Build history of the part. All positions in model axes, mm. Face numbers are marked on the shaded views. A direction names the side the tool comes from. Coordinates: 2 decimals unless noted, no trailing zeros. Order: outer loops, then holes, each group sorted by start corner. A loop starts at its lowest first (then second) coordinate and runs counter-clockwise, first axis right, second up. Notation, with made-up numbers: (76.5, 38) - (135.5, 38) arc R30 ccw to (135.5, 62) - close; hole circle Ø5 at (18, -12.75). An arc over 180 degrees is marked (long way). Write each question's results on one line, items separated by ' | '.
from build123d import *

# Parameters (mm, degrees)
SKETCH1_R               = 70
BOSS_EXTRUDE1_DEPTH     = 35
SKETCH2_R               = 62.5
BOSS_EXTRUDE2_DEPTH     = 150
FILLET1_R               = 20
SKETCH3_R               = 57.5
BOSS_EXTRUDE3_DEPTH     = 325
CUT_EXTRUDE1_DEPTH      = 15
CUT_EXTRUDE1_DEPTH_BACK = 15
FILLET2_R               = 10


with BuildPart() as part:
    # Sketch1 → Boss-Extrude1 (new body)
    with BuildSketch(Plane.XY):
        Circle(SKETCH1_R)
    extrude(amount=BOSS_EXTRUDE1_DEPTH)

    # Sketch2 → Boss-Extrude2 (add)
    with BuildSketch(Plane.XY):
        Circle(SKETCH2_R)
    extrude(amount=-BOSS_EXTRUDE2_DEPTH)

    # Fillet1
    # the kernel refuses this fillet: 20 mm, written as the material it adds along each edge
    with BuildSketch(Plane(origin=(0, 0, 0), x_dir=(1, 0, 0), z_dir=(0, -1, 0))) as fillet1_piece_1:
        with BuildLine():
            CenterArc((82.5, -15.612494996), FILLET1_R, 128.682187453, 51.317812547)
            Line((62.5, -15.612494996), (62.1, -15.612494996))
            Line((62.1, -15.612494996), (62.1, 0))
            Line((62.1, 0), (62.5, 0.4))
            ThreePointArc((62.5, 0.4), (66.25, 0.4), (69.75, 0.3122499))
            Line((69.75, 0.3122499), (70, 0))
        make_face()
    revolve(axis=Axis((0, 0, 0), (0, 0, 1)))

    # Sketch3 → Boss-Extrude3 (add)
    with BuildSketch(Plane.XY):
        Circle(SKETCH3_R)
    extrude(amount=BOSS_EXTRUDE3_DEPTH)

    # Sketch4 → Cut-Extrude1 (cut, two sides: drawn at the far end of the back side and taken through both)
    with BuildSketch(Plane(origin=(0, 0, 0), x_dir=(0, 0, -1), z_dir=(1, 0, 0)).offset(-CUT_EXTRUDE1_DEPTH_BACK)):
        Polygon((-240, 0), (-251.375, 273), (-60, 273), (-60, 0), (-60, -273), (-228.625, -273), align=None)
    extrude(amount=CUT_EXTRUDE1_DEPTH + CUT_EXTRUDE1_DEPTH_BACK, mode=Mode.SUBTRACT)

    # Fillet2
    fillet2_edges = [part.edges().sort_by_distance(p)[0] for p in [
        (-62.5, 0, -150),
    ]]
    fillet(fillet2_edges, radius=FILLET2_R)


solid = part.part
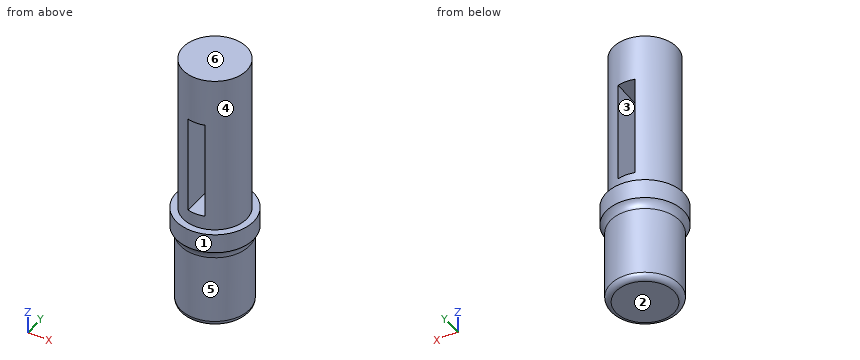
1. Band-saw the part on A-A on y = 0. Give the cut face in (x, z), then the cut area to 3 significant figures.
Solved:
outline: (-70, 0) arc R20 cw to (-62.5, -15.61) - (-62.5, -140) arc R10 ccw to (-52.5, -150) - (52.5, -150) arc R10 ccw to (62.5, -140) - (62.5, -15.61) arc R20 cw to (70, 0) - (70, 35) - (57.5, 35) - (57.5, 325) - (-57.5, 325) - (-57.5, 35) - (-70, 35) - close; hole (-15, 60) - (15, 60) - (15, 240) - (-15, 240) - close | area: 51,600 mm2
2. Band-saw the part on C-C on z = 206. Give the cut face in (x, y).
Solved:
outline: (-15, -55.51) - (-15, 55.51) arc R57.5 ccw to start; (15, -55.51) arc R57.5 ccw to (15, 55.51) - close
3. Two-plate mould, pull along X, no slides. Class the marked faces 1, 2 and 3: +X half, -X half, draft (parallel to the pull), parting line (faces both ways), or undercut.
Solved:
face 1: parting line | face 2: draft | face 3: undercut
4. Tool access for the marked faces 4, 5 and 6: list every direction of +Z, -Z, +X, -X, +Y, -Y with a clear straight run to the whole face (end or side of a thin tool).
Solved:
face 4: +Z | face 5: -Z | face 6: +Z, +X, -X, +Y, -Y
5. Band-saw the part on B-B on x = 0. Give the cut face in (y, z), then the cut area to 3 significant figures.
Solved:
outline: (-70, 0) arc R20 cw to (-62.5, -15.61) - (-62.5, -140) arc R10 ccw to (-52.5, -150) - (52.5, -150) arc R10 ccw to (62.5, -140) - (62.5, -15.61) arc R20 cw to (70, 0) - (70, 35) - (57.5, 35) - (57.5, 60) - (-57.5, 60) - (-57.5, 35) - (-70, 35) - close; (-57.5, 237.6) - (57.5, 242.4) - (57.5, 325) - (-57.5, 325) - close | area: 36,300 mm2
6. Drop flat-ended pins along their axis: pin 1 Ø6 at (x, z) = (-17, 46.5) entering from -Y; pin 2 Ø2 at (y, z) = (41.5, 131) entering from +X; pin 3 Ø1 at (y, z) = (-34.5, 98.5) entering from +X. Give the stop position or say it passes through.
Solved:
pin 1: stops at y = -55.77 | pin 2: stops at x = 40.82 | pin 3: stops at x = 46.37
7. Probe line 1 (Z direction, x = -6, y = 26); line 2 (X direction, y = 31.5, z = 112); line 3 (X direction, y = -2, z = 297). List the from-to ranges inside material, lowest first.
Solved:
line 1: z = -150 to 60, 241.08 to 325 | line 2: x = -48.1 to -15, 15 to 48.1 | line 3: x = -57.47 to 57.47
